Geometry check sheet. Reference: drawing and pictorial views, mm from the part's lowest x, y, z. A direction names the side the tool comes from. Give positions to 0.01 mm unless a question says otherwise; leave off trailing zeros. Write each loop counter-clockwise with the first axis right and the second up, starting at its lowest first coordinate (ties: lowest second). Pieces come first, ordered by that corner, then holes. Notation, with made-up numbers: (-19.75, 31.25) - (-2.75, 31.25) arc R24 cw to (-2.75, 60.25) - close; hole circle Ø6 at (9, 23.25). An arc over 180 degrees is marked (long way). Put each result on its own line as item: value.
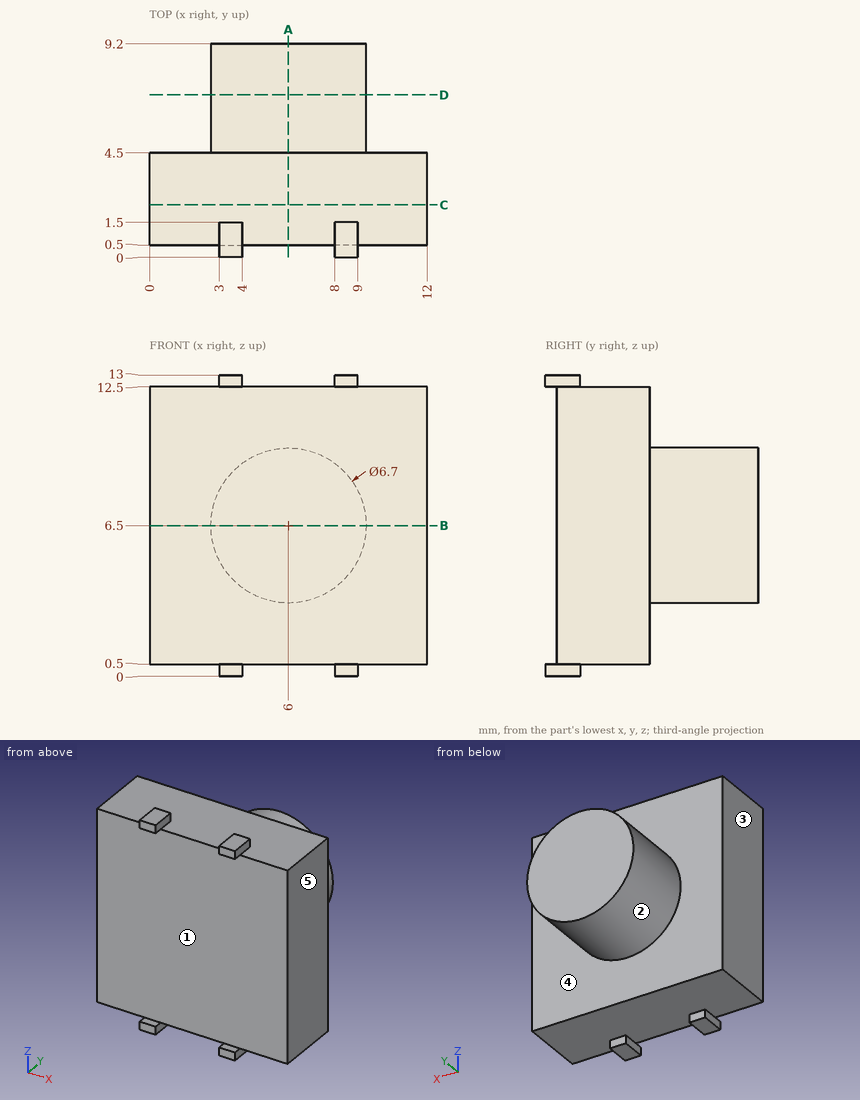
Q1. Section check B-B, the plane z = 6.5. Record the cut outline in (x, y).
Answers follow:
outline: (0, 0.5) - (12, 0.5) - (12, 4.5) - (9.35, 4.5) - (9.35, 9.2) - (2.65, 9.2) - (2.65, 4.5) - (0, 4.5) - close
Q2. Scan lines: line 1 along Y through (x, z) = (4.25, 8.25); line 2 along Y through (x, z) = (3.75, 3.25); line 3 along Z through (x, y) = (1.25, 4). Record each from-to range of solid material in increasing order.
Answers follow:
line 1: y = 0.5 to 9.2
line 2: y = 0.5 to 4.5
line 3: z = 0.5 to 12.5
Q3. Go/stop test with a flat-tipped pin: pin 1 Ø1.5 at (x, y) = (5.5, 2.5) entering from +Z. Record where the tip stops, or that it passes through.
Answers follow:
pin 1: stops at z = 12.5
Q4. Section check D-D, the plane y = 7. Record the cut outline in (x, z).
Answers follow:
outline: circle Ø6.7 at (6, 6.5)
Q5. Section check A-A, the plane x = 6. Record the cut outline in (y, z).
Answers follow:
outline: (0.5, 0.5) - (4.5, 0.5) - (4.5, 3.15) - (9.2, 3.15) - (9.2, 9.85) - (4.5, 9.85) - (4.5, 12.5) - (0.5, 12.5) - close
Q6. Release check for a two-part mould opening along Z. For the marked faces 1, 2 and 3 record: released by +Z, released by -Z, zero draft, split by the parting line, or undercut.
Answers follow:
face 1: undercut
face 2: split by the parting line
face 3: zero draft
Q7. Section check C-C, the plane y = 2.25. Record the cut outline in (x, z).
Answers follow:
outline: (0, 0.5) - (12, 0.5) - (12, 12.5) - (0, 12.5) - close
Q8. Set-up check for the marked faces 4 and 5: record each of +Z, -Z, +X, -X, +Y, -Y from which the full face is reachable in a straight line by a thin tool's end or side.
Answers follow:
face 4: +Y
face 5: +Z, -Z, +X, +Y, -Y
